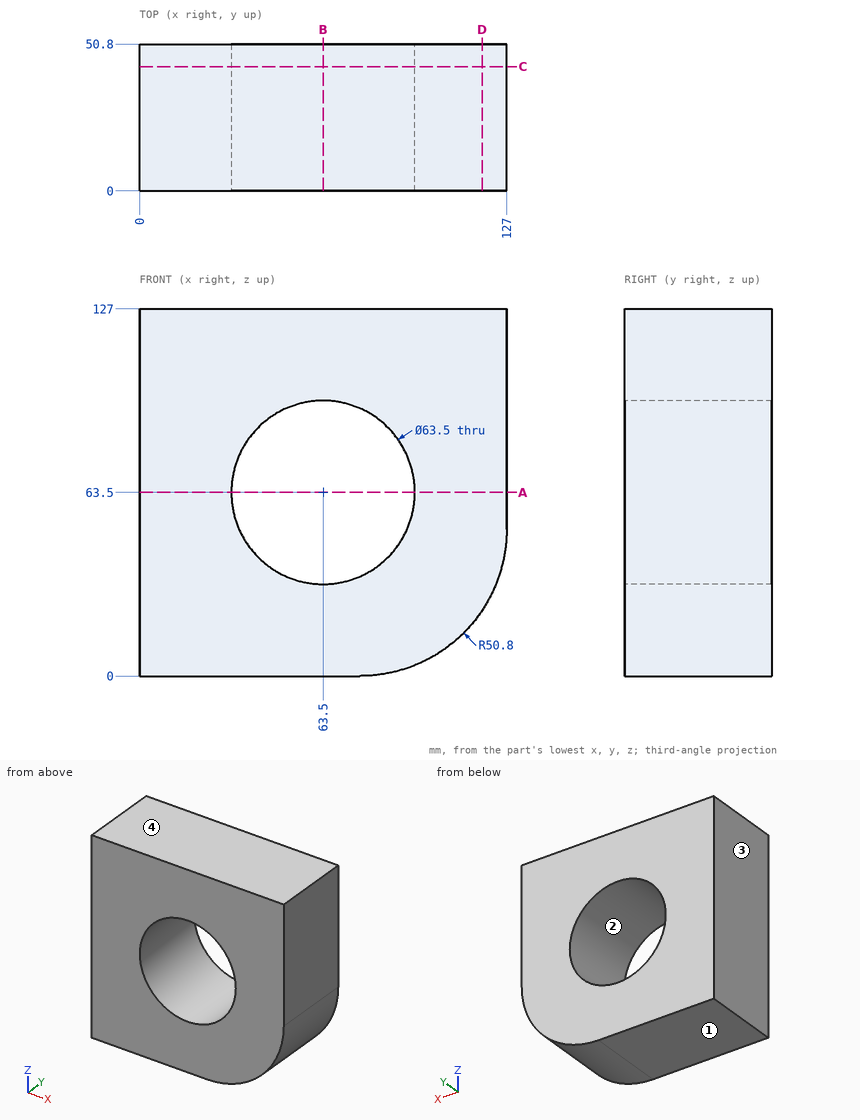
Here's the drawing with two shaded views (mm, measured from the low corner). I have some questions. Coordinates: 2 decimals unless noted, no trailing zeros. Write each loop counter-clockwise with the first axis right and the second up, starting at its lowest first coordinate (ties: lowest second). Pieces come first, ordered by that corner, then holes. Notation, with made-up numbers: M 49,27.5 L 104,27.5 A15 cw 104,53.5 Z; hole C 13.25,12 d6. An arc over 180 degrees is marked long. Answer as CSV lines item,"result".
Item 1: Imagine slicing it at A-A on z = 63.5. List the corners of the cut face in (x, y) for me, plus the area to 3 significant figures.
Geometry results:
outline,"M 0,0 L 31.75,0 L 31.75,50.8 L 0,50.8 Z; M 95.25,0 L 127,0 L 127,50.8 L 95.25,50.8 Z"
area,"3,230 mm2"
Item 2: We'd pull the mould along Z, two halves only. Please class the marked faces 1, 2, 3 and 4: +Z half, -Z half, draft (parallel to the pull), parting line (faces both ways), or undercut.
Geometry results:
face 1,"-Z half"
face 2,"undercut"
face 3,"draft"
face 4,"+Z half"
Item 3: Imagine slicing it at C-C on y = 43. List the corners of the cut face in (x, z) for me.
Geometry results:
outline,"M 0,0 L 76.2,0 A50.8 ccw 127,50.8 L 127,127 L 0,127 Z; hole C 63.5,63.5 d63.5"
Item 4: Please list where these lines run through material, in increasing order: line 1 along Z through (x, y) = (63, 37); line 2 along Z through (x, y) = (71.5, 20.5).
Geometry results:
line 1,"z = 0 to 31.75, 95.25 to 127"
line 2,"z = 0 to 32.77, 94.23 to 127"
Item 5: Imagine slicing it at B-B on x = 63.5. List the corners of the cut face in (y, z) for me, plus the area to 3 significant figures.
Geometry results:
outline,"M 0,0 L 50.8,0 L 50.8,31.75 L 0,31.75 Z; M 0,95.25 L 50.8,95.25 L 50.8,127 L 0,127 Z"
area,"3,230 mm2"
Item 6: I'm going to push flat-ended pins straight in: P1, Ø3, axis at y = 33, z = 90, coming from the -X side; P2, Ø2, axis at x = 97.5, y = 45, coming from the -Z side; P3, Ø10, axis at x = 110.5, y = 13, coming from the -Z side. Where does each tip first touch, or does it pass through?
Geometry results:
P1,"stops at x = 0"
P2,"stops at z = 4.23"
P3,"stops at z = 9.3"
Item 7: Imagine slicing it at D-D on x = 118.5. List the corners of the cut face in (y, z) for me.
Geometry results:
outline,"M 0,22.67 L 50.8,22.67 L 50.8,127 L 0,127 Z"
